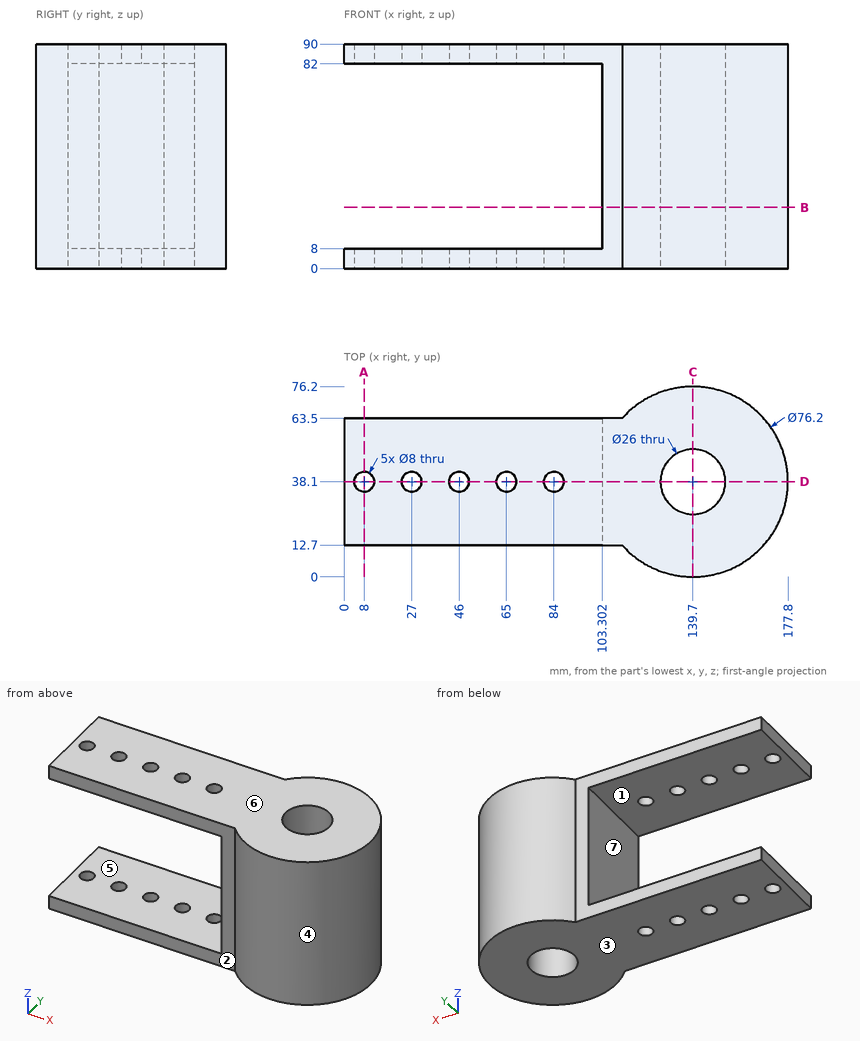
Source: three-view drawing plus pictorial views. Frame: mm from the lowest corner of the part. A direction names the side the tool comes from. Round coordinates to 2 decimals unless told otherwise and drop trailing zeros. Loops run counter-clockwise (first coordinate to the right, second up) from the corner with the lowest first, then second, coordinate; pieces in that order, holes last.
1. Section query B-B on z = 24.5. Output: boundary loops of the cut face in (x, y).
2. Section query A-A on x = 8. Output: boundary loops of the cut face in (y, z).
3. Access query for the marked faces 1, 2 and 3. Directions: +Z, -Z, +X, -X, +Y, -Y. A direction counts if a zero-diameter tool reaches every point of the face in a straight line with its end or side. Return the directions, or none.
4. Contact query for flat-ended pins moving along their axis: pin 1 (1 mm diameter, centred on y = 34.5, z = 60.5, fed in from -X); pin 2 (6 mm diameter, centred on y = 9, z = 73, fed in from +X); pin 3 (5 mm diameter, centred on x = 8, y = 38.1, fed in from -Z) (3 decimals); pin 4 (13 mm diameter, centred on x = 65, y = 38.1, fed in from -Z). Output: stop coordinate, or through.
5. Section query D-D on y = 38.1. Give the number of separate pieces and of enclosed holes in the cut face, and give its area (3 significant figures).
6. Mould query, pull axis Z, two halves, no side actions, for the marked faces 4, 5, 6 and 7. Classes: released by +Z, released by -Z, zero draft, split by the parting line, or undercut.
7. Section query C-C on x = 139.7. Output: boundary loops of the cut face in (y, z), and give its area (3 significant figures).
8. Ray query, L1, parallel to Y at x = 139.7, z = 39; L2, parallel to Z at x = 23, y = 53.5; L3, parallel to Y at x = 8, z = 88.25. Return the intervals inside material, ascending.
Answers below:
1. outline: (103.3, 12.7) - (111.3, 12.7) arc R38.1 ccw (long way) to (111.3, 63.5) - (103.3, 63.5) - close; hole circle Ø26 at (139.7, 38.1)
2. outline: (12.7, 0) - (34.1, 0) - (34.1, 8) - (12.7, 8) - close; (12.7, 82) - (34.1, 82) - (34.1, 90) - (12.7, 90) - close; (42.1, 0) - (63.5, 0) - (63.5, 8) - (42.1, 8) - close; (42.1, 82) - (63.5, 82) - (63.5, 90) - (42.1, 90) - close
3. face 1: -X, +Y, -Y
3. face 2: +Z, -Z, -X, -Y
3. face 3: -Z, +X, -X, +Y, -Y
4. pin 1: stops at x = 103.3
4. pin 2: stops at x = 167.46
4. pin 3: passes through
4. pin 4: stops at z = 0
5. separate pieces: 12
5. enclosed holes: 0
5. area: 5,380 mm2
6. face 4: zero draft
6. face 5: undercut
6. face 6: released by +Z
6. face 7: undercut
7. outline: (0, 0) - (25.1, 0) - (25.1, 90) - (0, 90) - close; (51.1, 0) - (76.2, 0) - (76.2, 90) - (51.1, 90) - close
7. area: 4,520 mm2
8. L1: y = 0 to 25.1, 51.1 to 76.2
8. L2: z = 0 to 8, 82 to 90
8. L3: y = 12.7 to 34.1, 42.1 to 63.5
